Work out the finished part from the listing and answer in its coordinate system (mm). A direction names the side the tool comes from. Give positions to 0.01 mm unless a question says otherwise; leave off trailing zeros. Order: outer loops, then holes, each group sorted by start corner. A loop starts at its lowest first (then second) coordinate and runs counter-clockwise, first axis right, second up. Notation, with made-up numbers: (-8, -14.5) -> (-1, -14.5) arc R19 cw to (-1, -0.5) -> close; hole circle Ø5 at (40, 73). An arc over 180 degrees is marked (long way). Answer as CSV lines item,"result". Start each with the question number.
1. For a pull along Z with two mould halves and no side action, classify faces 1 (the flat face through (95.3, 5, -18.5)), 2 (the flat face through (106, 3, -15)), 3 (the flat face through (91, 1, -40)), 4 (the cylindrical face through (156.614, 1.479, -4.425)) as released by +Z, released by -Z, zero draft, split by the parting line, or undercut.
2. Flat-ended cylindrical pins translate along their axes: pin 1 (2 mm diameter, centred on y = 1.5, z = -13, fed in from +X); pin 2 (0.6 mm diameter, centred on x = 108.5, y = 3.5, fed in from +Z); pin 3 (3 mm diameter, centred on x = 72.5, z = -14.5, fed in from +Y). Find the tip coordinate at first contact, or state that the pin passes through.
3. A cutting plane is placed at C-C (y = 1). Give the vertices of the cut face in (x, z).
4. A cutting plane is placed at A-A (z = -35). Give the vertices of the cut face in (x, y), then the cut area to 3 significant figures.
5. A cutting plane is placed at B-B (x = 5). Give the vertices of the cut face in (y, z).
6. Find the intervals of material crossed by L1, parallel to X at y = 4, z = -19.5 (3 decimals); L2, parallel to Y at x = 46, z = -22; L3, parallel to Z at x = 5, y = 1.2, in increasing order.
7. For faces 5 (the flat face through (74, 3, -22)), 6 (the cylindrical face through (5.325, 1.479, -33.536)), determine the directions among +Z, -Z, +X, -X, +Y, -Y from which every point of the face is accessible in a straight line to the end or side of a thin tool.
8. A cutting plane is placed at D-D (z = -5). Give the vertices of the cut face in (x, y), then the cut area to 3 significant figures.
Autodesk Inventor part; units mm, degrees
ref_plane "YZ Plane" through (0, 0, 0) normal (1, 0, 0) x (0, 1, 0)
ref_plane "XZ Plane" through (0, 0, 0) normal (0, 1, 0) x (-1, 0, 0)
ref_plane "XY Plane" through (0, 0, 0) normal (0, 0, 1) x (1, 0, 0)
sketch "스케치1" plane through (0, 0, 0) normal (0, 1, 0) x (-1, 0, 0)
  line L0 (-25, 0) -> (-155, 0)
  line L1 (-180, -25) -> (-180, -40)
  line L2 (-180, -40) -> (0, -40)
  line L3 (0, -40) -> (0, -25)
  arc A0 (0, -25) -> (-25, 0) centre (-25, -25) ccw
  arc A1 (-155, 0) -> (-180, -25) centre (-155, -25) ccw
  circle A2 centre (-5, -35) radius 1.5
  circle A3 centre (-5, -35) radius 2.5
  circle A4 centre (-5, -22) radius 1.5
  circle A5 centre (-5, -22) radius 2.5
  circle A6 centre (-22, -5) radius 1.5
  circle A7 centre (-22, -5) radius 2.5
  line L4 (-90, -40) -> (-90, 0)
  circle A8 centre (-90, -35) radius 2.5
  circle A9 centre (-90, -5) radius 2.5
  circle A10 centre (-47.5, -35) radius 2.5
  circle A11 centre (-175, -35) radius 1.5
  circle A12 centre (-175, -35) radius 2.5
  circle A13 centre (-175, -22) radius 1.5
  circle A14 centre (-175, -22) radius 2.5
  circle A15 centre (-158, -5) radius 1.5
  circle A16 centre (-158, -5) radius 2.5
  circle A17 centre (-132.5, -35) radius 2.5
  point P0 (0, 0)
  point P1 (-180, 0)
  dimension "d0" = 180
  dimension "d1" = 40
  dimension "d2" = 25
  dimension "d3" = 3
  dimension "d4" = 5
  dimension "d5" = 3
  dimension "d6" = 5
  dimension "d7" = 3
  dimension "d8" = 5
  dimension "d9" = 5
  dimension "d10" = 5
  dimension "d11" = 5
  dimension "d12" = 5
  dimension "d13" = 5
  dimension "d14" = 5
  dimension "d15" = 5
  dimension "d16" = 5
  dimension "d17" = 5
  dimension "d18" = 85
  dimension "d19" = 42.5
  dimension "d20" = 3
  dimension "d21" = 3
extrude "돌출1" add sketch "스케치1" along normal blind 3 contours A0 L3 L2 L4 A8 A9 L0 | L4 A9 A8 L2 L1 A1 L0 | A9 L4 | L4 A9 | A8 L4 | L4 A8 | A3 | A4 | A5 | A7 | A10 | A12 | A13 | A14 | A16 | A17
sketch "스케치2" plane through (0, 3, 0) normal (0, 1, 0) x (1, 0, 0)
  line L0 (113.9465, 8.0671) -> (66.0535, 8.0671) construction
  line L1 (66.0535, 8.0671) -> (66.0535, 31.9329) construction
  line L2 (66.0535, 31.9329) -> (113.9465, 31.9329) construction
  line L3 (113.9465, 31.9329) -> (113.9465, 8.0671) construction
  line L4 (0, 40) -> (0, 25)
  line L5 (180, 40) -> (0, 40)
  spline S0 degree 2 poles (99.2788, 14.4529) (99.2788, 15.7494) (100.2026, 18.0833) (101.0292, 18.8937) knots 0 0 0 1 2 2 2
  spline S1 degree 2 poles (101.0292, 18.8937) (102.0664, 19.9148) (104.8703, 20.9682) (107.0097, 20.9682) knots 0 0 0 1 2 2 2
  line L6 (107.0097, 20.9682) -> (109.2626, 20.9682)
  line L7 (109.2626, 20.9682) -> (109.2626, 28.4237)
  line L8 (109.2626, 28.4237) -> (111.9206, 28.4237)
  line L9 (111.9206, 28.4237) -> (111.9206, 8.4237)
  line L10 (111.9206, 8.4237) -> (106.8963, 8.4237)
  spline S2 degree 2 poles (106.8963, 8.4237) (105.1135, 8.4237) (102.6175, 9.0071) (101.6613, 9.6717) knots 0 0 0 1 2 2 2
  spline S3 degree 2 poles (101.6613, 9.6717) (100.5429, 10.4334) (99.2788, 12.7835) (99.2788, 14.4529) knots 0 0 0 1 2 2 2
  spline S4 degree 2 poles (102.0502, 14.5339) (102.0502, 13.4966) (102.7634, 11.9731) (103.4927, 11.4869) knots 0 0 0 1 2 2 2
  spline S5 degree 2 poles (103.4927, 11.4869) (104.1248, 11.0655) (105.8104, 10.7251) (107.0583, 10.7251) knots 0 0 0 1 2 2 2
  line L11 (107.0583, 10.7251) -> (109.2626, 10.7251)
  line L12 (109.2626, 10.7251) -> (109.2626, 18.6992)
  line L13 (109.2626, 18.6992) -> (107.4473, 18.6992)
  spline S6 degree 2 poles (107.4473, 18.6992) (105.8266, 18.6992) (103.8331, 18.1806) (103.1848, 17.4999) knots 0 0 0 1 2 2 2
  spline S7 degree 2 poles (103.1848, 17.4999) (102.5851, 16.9002) (102.0502, 15.4901) (102.0502, 14.5339) knots 0 0 0 1 2 2 2
  spline S8 degree 2 poles (88.9384, 28.7802) (90.8833, 28.7802) (94.1734, 27.4674) (95.3728, 26.1546) knots 0 0 0 1 2 2 2
  spline S9 degree 2 poles (95.3728, 26.1546) (96.5721, 24.858) (97.8849, 20.9682) (97.8849, 18.4399) knots 0 0 0 1 2 2 2
  spline S10 degree 2 poles (97.8849, 18.4399) (97.8849, 15.9277) (96.6045, 12.2) (95.389, 10.8224) knots 0 0 0 1 2 2 2
  spline S11 degree 2 poles (95.389, 10.8224) (94.1896, 9.4772) (90.9157, 8.0671) (88.8898, 8.0671) knots 0 0 0 1 2 2 2
  spline S12 degree 2 poles (88.8898, 8.0671) (87.8849, 8.0671) (86.1183, 8.3588) (85.3728, 8.5858) knots 0 0 0 1 2 2 2
  spline S13 degree 2 poles (85.3728, 8.5858) (84.7245, 8.7964) (83.3793, 9.3961) (82.7147, 9.7527) knots 0 0 0 1 2 2 2
  line L14 (82.7147, 9.7527) -> (82.7147, 12.9618)
  line L15 (82.7147, 12.9618) -> (82.9254, 12.9618)
  spline S14 degree 2 poles (82.9254, 12.9618) (83.282, 12.6376) (84.3841, 11.73) (85.1783, 11.2924) knots 0 0 0 1 2 2 2
  spline S15 degree 2 poles (85.1783, 11.2924) (85.94, 10.871) (87.7391, 10.3362) (88.906, 10.3362) knots 0 0 0 1 2 2 2
  spline S16 degree 2 poles (88.906, 10.3362) (90.1864, 10.3362) (92.4716, 11.3896) (93.3306, 12.3945) knots 0 0 0 1 2 2 2
  spline S17 degree 2 poles (93.3306, 12.3945) (94.1734, 13.4156) (95.1135, 16.5112) (95.1135, 18.4399) knots 0 0 0 1 2 2 2
  spline S18 degree 2 poles (95.1135, 18.4399) (95.1135, 20.4982) (94.1248, 23.4642) (93.2658, 24.4853) knots 0 0 0 1 2 2 2
  spline S19 degree 2 poles (93.2658, 24.4853) (92.423, 25.4739) (90.1702, 26.4788) (88.906, 26.4788) knots 0 0 0 1 2 2 2
  spline S20 degree 2 poles (88.906, 26.4788) (87.7553, 26.4788) (85.7942, 25.9115) (85.0324, 25.4901) knots 0 0 0 1 2 2 2
  spline S21 degree 2 poles (85.0324, 25.4901) (84.3031, 25.0687) (83.2172, 24.1935) (82.9092, 23.8856) knots 0 0 0 1 2 2 2
  line L16 (82.9092, 23.8856) -> (82.7147, 23.8856)
  line L17 (82.7147, 23.8856) -> (82.7147, 27.0623)
  spline S22 degree 2 poles (82.7147, 27.0623) (83.3793, 27.3702) (84.5462, 27.9375) (85.3728, 28.1968) knots 0 0 0 1 2 2 2
  spline S23 degree 2 poles (85.3728, 28.1968) (86.248, 28.4885) (87.7391, 28.7802) (88.9384, 28.7802) knots 0 0 0 1 2 2 2
  spline S24 degree 2 poles (66.6694, 22.2811) (66.6694, 23.7721) (67.8039, 26.0574) (68.7439, 26.8029) knots 0 0 0 1 2 2 2
  spline S25 degree 2 poles (68.7439, 26.8029) (69.8784, 27.6781) (72.4554, 28.4237) (74.4976, 28.4237) knots 0 0 0 1 2 2 2
  line L18 (74.4976, 28.4237) -> (80.235, 28.4237)
  line L19 (80.235, 28.4237) -> (80.235, 8.4237)
  line L20 (80.235, 8.4237) -> (74.9352, 8.4237)
  spline S26 degree 2 poles (74.9352, 8.4237) (72.7958, 8.4237) (70.6564, 8.6992) (69.684, 9.234) knots 0 0 0 1 2 2 2
  spline S27 degree 2 poles (69.684, 9.234) (68.5981, 9.8013) (67.6094, 11.6652) (67.6094, 12.9293) knots 0 0 0 1 2 2 2
  spline S28 degree 2 poles (67.6094, 12.9293) (67.6094, 14.3394) (69.1005, 16.576) (70.4133, 17.2081) knots 0 0 0 1 2 2 2
  line L21 (70.4133, 17.2081) -> (70.4133, 17.3054)
  spline S29 degree 2 poles (70.4133, 17.3054) (68.6305, 17.7916) (66.6694, 20.3686) (66.6694, 22.2811) knots 0 0 0 1 2 2 2
  spline S30 degree 2 poles (69.4408, 22.3945) (69.4408, 21.26) (70.0891, 19.8013) (71.0616, 19.2827) knots 0 0 0 1 2 2 2
  spline S31 degree 2 poles (71.0616, 19.2827) (71.6937, 18.9585) (73.1848, 18.764) (74.5624, 18.764) knots 0 0 0 1 2 2 2
  line L22 (74.5624, 18.764) -> (77.577, 18.764)
  line L23 (77.577, 18.764) -> (77.577, 26.1546)
  line L24 (77.577, 26.1546) -> (75.4214, 26.1546)
  spline S32 degree 2 poles (75.4214, 26.1546) (73.671, 26.1546) (71.6613, 25.8305) (70.8833, 25.3118) knots 0 0 0 1 2 2 2
  spline S33 degree 2 poles (70.8833, 25.3118) (70.1378, 24.777) (69.4408, 23.448) (69.4408, 22.3945) knots 0 0 0 1 2 2 2
  spline S34 degree 2 poles (70.3809, 13.3021) (70.3809, 12.589) (70.8671, 11.5193) (71.4019, 11.2114) knots 0 0 0 1 2 2 2
  spline S35 degree 2 poles (71.4019, 11.2114) (72.0502, 10.8548) (73.6224, 10.6927) (75.0324, 10.6927) knots 0 0 0 1 2 2 2
  line L25 (75.0324, 10.6927) -> (77.577, 10.6927)
  line L26 (77.577, 10.6927) -> (77.577, 16.5436)
  line L27 (77.577, 16.5436) -> (74.5624, 16.5436)
  spline S36 degree 2 poles (74.5624, 16.5436) (73.3144, 16.5436) (72.1313, 16.2843) (71.4992, 15.8791) knots 0 0 0 1 2 2 2
  spline S37 degree 2 poles (71.4992, 15.8791) (70.8833, 15.4901) (70.3809, 14.2422) (70.3809, 13.3021) knots 0 0 0 1 2 2 2
  point P0 (0, 0)
  point P1 (90, 8.0671)
  point P2 (66.0535, 20)
  dimension "d24" = 90
  dimension "d25" = 20
extrude "돌출2" add sketch "스케치2" along normal blind 2
properties part number "pcb"
Answer sheet:
1,face 1,"zero draft"
1,face 2,"undercut"
1,face 3,"released by -Z"
1,face 4,"undercut"
2,pin 1,"stops at x = 177.45"
2,pin 2,"stops at z = -8.42"
2,pin 3,"stops at y = 3"
3,outline,"(0, -40) -> (180, -40) -> (180, -25) arc R25 ccw to (155, 0) -> (25, 0) arc R25 ccw to (0, -25) -> close; hole circle Ø3 at (5, -35); hole circle Ø3 at (22, -5); hole circle Ø3 at (158, -5); hole circle Ø3 at (175, -35)"
4,outline,"(0, 0) -> (3.5, 0) -> (3.5, 3) -> (0, 3) -> close; (6.5, 0) -> (173.5, 0) -> (173.5, 3) -> (6.5, 3) -> close; (176.5, 0) -> (180, 0) -> (180, 3) -> (176.5, 3) -> close"
4,area,"522 mm^2"
5,outline,"(0, -40) -> (3, -40) -> (3, -36.5) -> (0, -36.5) -> close; (0, -33.5) -> (3, -33.5) -> (3, -10) -> (0, -10) -> close"
6,L1,"x = 67.366 to 70.696, 77.577 to 80.235, 95.078 to 97.855, 101.735 to 111.921"
6,L2,"y = 0 to 3"
6,L3,"z = -40 to -36.5, -33.5 to -10"
7,face 5,"+Y"
7,face 6,"+Y, -Y"
8,outline,"(10, 0) -> (20.5, 0) -> (20.5, 3) -> (10, 3) -> close; (23.5, 0) -> (156.5, 0) -> (156.5, 3) -> (23.5, 3) -> close; (159.5, 0) -> (170, 0) -> (170, 3) -> (159.5, 3) -> close"
8,area,"462 mm^2"
